Autodesk Inventor part; units mm, degrees
ref_plane "YZ Plane" through (0, 0, 0) normal (1, 0, 0) x (0, 1, 0)
ref_plane "XZ Plane" through (0, 0, 0) normal (0, 1, 0) x (-1, 0, 0)
ref_plane "XY Plane" through (0, 0, 0) normal (0, 0, 1) x (1, 0, 0)
sketch "Sketch1" plane through (0, 0, 0) normal (0, 1, 0) x (-1, 0, 0)
  line L0 (7.6, 58.6) -> (-7.6, 58.6)
  line L1 (-7.6, 58.6) -> (-7.6, -58.6)
  line L2 (-7.6, -58.6) -> (7.6, -58.6)
  line L3 (7.6, -58.6) -> (7.6, 58.6)
  line L4 (7.6, 58.6) -> (-7.6, -58.6) construction
  line L5 (-7.6, 58.6) -> (7.6, -58.6) construction
  line L6 (10.6, 61.6) -> (-10.6, 61.6)
  line L7 (-10.6, 61.6) -> (-10.6, -61.6)
  line L8 (-10.6, -61.6) -> (10.6, -61.6)
  line L9 (10.6, -61.6) -> (10.6, 61.6)
  point P0 (0, 0)
  dimension "d0" = 15.2
  dimension "d1" = 117.2
  dimension "d2" = 3
extrude "Extrusion1" add sketch "Sketch1" along normal blind 35
sketch "Sketch2" plane through (0, 0, 0) normal (0, -1, 0) x (1, 0, 0)
  circle A0 centre (15.6, 56.6) radius 2.25
  line L0 (10.6, 61.6) -> (10.6, -61.6)
  line L1 (-10.6, 61.6) -> (10.6, 61.6)
  line L2 (10.6, 0) -> (40.0952, 0)
  line L3 (10.6, -61.6) -> (-10.6, -61.6)
  line L4 (0, -61.6) -> (0, -71.4925)
  line L5 (10.6, 61.6) -> (20.6, 61.6)
  line L6 (20.6, 61.6) -> (20.6, 51.6)
  line L7 (20.6, 51.6) -> (10.6, 51.6)
  line L8 (10.6, 51.6) -> (10.6, 61.6)
  line L9 (-10.6, 61.6) -> (10.6, 61.6)
  line L10 (10.6, 61.6) -> (10.6, -61.6)
  line L11 (10.6, -61.6) -> (-10.6, -61.6)
  line L12 (-10.6, -61.6) -> (-10.6, 61.6)
  circle A1 centre (15.6, -56.6) radius 2.25
  line L13 (10.6, -61.6) -> (20.6, -61.6)
  line L14 (20.6, -61.6) -> (20.6, -51.6)
  line L15 (20.6, -51.6) -> (10.6, -51.6)
  line L16 (10.6, -51.6) -> (10.6, -61.6)
  circle A2 centre (-15.6, 56.6) radius 2.25
  line L17 (-10.6, 61.6) -> (-20.6, 61.6)
  line L18 (-20.6, 61.6) -> (-20.6, 51.6)
  line L19 (-20.6, 51.6) -> (-10.6, 51.6)
  line L20 (-10.6, 51.6) -> (-10.6, 61.6)
  line L21 (-20.6, -51.6) -> (-10.6, -51.6)
  circle A3 centre (-15.6, -56.6) radius 2.25
  line L22 (-10.6, -61.6) -> (-20.6, -61.6)
  line L23 (-20.6, -61.6) -> (-20.6, -51.6)
  line L24 (-10.6, -51.6) -> (-10.6, -61.6)
  point P0 (0, 0)
  dimension "d5" = 4.5
  dimension "d6" = 5
  dimension "d7" = 5
  dimension "d8" = 5
  dimension "d9" = 5
extrude "Extrusion2" add sketch "Sketch2" along normal blind 3
properties part number "HDD_fastening"
The listing builds one solid part. Answer for the finished solid, in the listing's coordinates (mm). A direction names the side the tool comes from. Round coordinates to 2 decimals unless told otherwise and drop trailing zeros. Write each loop counter-clockwise with the first axis right and the second up, starting at its lowest first coordinate (ties: lowest second). Pieces come first, ordered by that corner, then holes. Notation, with made-up numbers: M 70.5,30 L 128.5,30 A16 ccw 128.5,37 Z; hole C 9,-30 d9. An arc over 180 degrees is marked long. Write each question's results on one line, items separated by ' | '. Start each with the question number.
(1) For faces 1 (the flat face through (-16, -1, 51.6)), 2 (the flat face through (-16, 0, -54)), 3 (the flat face through (0, 16, 61.6)), 4 (the flat face through (-7.6, 17, -1)), 5 (the flat face through (16, -1, -51.6)), determine the directions among +Z, -Z, +X, -X, +Y, -Y from which every point of the face is accessible in a straight line to the end or side of a thin tool.
(2) Find the intervals of material crossed by line 1 (Z direction, x = -15.6, y = -2.2); line 2 (X direction, y = 21, z = 4); line 3 (Z direction, x = 5, y = 6), in increasing order.
(3) The part is cut by section B-B, the plane x = -15.6. Write down the section's boundary in (y, z).
(4) The part is cut by section D-D, the plane z = -14. Write down the section's boundary in (x, y).
(5) Determine the mould class of faces 6 (the flat face through (-20.6, -1, -57)), 7 (the cylindrical face through (-17.386, -1.479, -55.231)), 8 (the flat face through (16, 0, -54)) for opening direction X: +X half, -X half, draft (parallel to the pull), parting line (faces both ways), or undercut.
(6) The part is cut by section C-C, the plane y = 29. Write down the section's boundary in (x, z), and give its area (3 significant figures).
(7) The part is cut by section A-A, the plane z = 56.6. Write down the section's boundary in (x, y), and give its area (3 significant figures).
(8) Each of these flat-tipped pins is pushed along its axis until it touches: P1, Ø3, axis at x = 13.5, z = -56, coming from the +Y side; P2, Ø1, axis at y = 6.5, z = 29, coming from the +X side; P3, Ø4, axis at x = -15.6, z = -56.6, coming from the +Y side; P4, Ø19, axis at y = 12.5, z = 24.5, coming from the -X side. Where does it stop, or does it pass through?
Worked answers:
1) face 1: -X, +Y, -Y | face 2: +Z, -Z, -X, +Y | face 3: +Z, +X, -X, +Y, -Y | face 4: +Y | face 5: +X, +Y, -Y
2) line 1: z = -61.6 to -58.85, -54.35 to -51.6, 51.6 to 54.35, 58.85 to 61.6 | line 2: x = -10.6 to -7.6, 7.6 to 10.6 | line 3: z = -61.6 to -58.6, 58.6 to 61.6
3) outline: M -3,-61.6 L 0,-61.6 L 0,-58.85 L -3,-58.85 Z; M -3,-54.35 L 0,-54.35 L 0,-51.6 L -3,-51.6 Z; M -3,51.6 L 0,51.6 L 0,54.35 L -3,54.35 Z; M -3,58.85 L 0,58.85 L 0,61.6 L -3,61.6 Z
4) outline: M -10.6,-3 L 10.6,-3 L 10.6,35 L 7.6,35 L 7.6,0 L -7.6,0 L -7.6,35 L -10.6,35 Z
5) face 6: -X half | face 7: undercut | face 8: draft
6) outline: M -10.6,-61.6 L 10.6,-61.6 L 10.6,61.6 L -10.6,61.6 Z; hole M -7.6,-58.6 L 7.6,-58.6 L 7.6,58.6 L -7.6,58.6 Z | area: 830 mm²
7) outline: M -20.6,-3 L -17.85,-3 L -17.85,0 L -20.6,0 Z; M -13.35,-3 L 13.35,-3 L 13.35,0 L 10.6,0 L 10.6,35 L 7.6,35 L 7.6,0 L -7.6,0 L -7.6,35 L -10.6,35 L -10.6,0 L -13.35,0 Z; M 17.85,-3 L 20.6,-3 L 20.6,0 L 17.85,0 Z | area: 307 mm²
8) P1: stops at y = 0 | P2: stops at x = 10.6 | P3: passes through | P4: stops at x = -10.6
